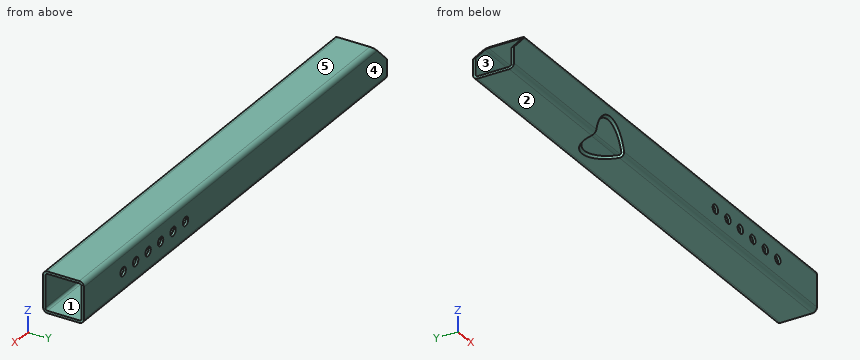
```python
from build123d import *

# Parameters (mm, degrees)
EL_MENT_M_CANO_SOUD_1_DEPTH = 850
ESQUISSE3_R                 = 7.5
ENL_V_MAT_EXTRU_2_DEPTH     = 90
ENL_V_MAT_EXTRU_3_DEPTH     = 71
ESQUISSE6_R                 = 40.75
ENL_V_MAT_EXTRU_4_DEPTH     = 90


with BuildPart() as part:
    # tube carré1 → Elément mécano-soudé1 (new body)
    with BuildSketch(Plane.YZ.offset(-425)):
        with BuildLine():
            Line((-27, 35), (27, 35))
            ThreePointArc((27, 35), (32.656854249, 32.656854249), (35, 27))
            Line((35, 27), (35, -27))
            ThreePointArc((35, -27), (32.656854249, -32.656854249), (27, -35))
            Line((27, -35), (-27, -35))
            ThreePointArc((-27, -35), (-32.656854249, -32.656854249), (-35, -27))
            Line((-35, -27), (-35, 27))
            ThreePointArc((-35, 27), (-32.656854249, 32.656854249), (-27, 35))
        make_face()
        with BuildLine():
            Line((-27, 31), (27, 31))
            ThreePointArc((27, 31), (29.828427336, 29.828426914), (31, 26.999999403))
            Line((31, 26.999999403), (31, -26.999999403))
            ThreePointArc((31, -26.999999403), (29.828427336, -29.828426914), (27, -31))
            Line((27, -31), (-27, -31))
            ThreePointArc((-27, -31), (-29.828427336, -29.828426914), (-31, -26.999999403))
            Line((-31, -26.999999403), (-31, 26.999999403))
            ThreePointArc((-31, 26.999999403), (-29.828427336, 29.828426914), (-27, 31))
        make_face(mode=Mode.SUBTRACT)
    extrude(amount=EL_MENT_M_CANO_SOUD_1_DEPTH)

    # Esquisse3 → Enlèv. mat.-Extru.2 (cut)
    with BuildSketch(Plane(origin=(0, 35, 0), x_dir=(1, 0, 0), z_dir=(0, 1, 0))):
        with Locations(Location((315, 0, 0), (0, 0, 270))):  # turned: the seam where the file's is
            Circle(ESQUISSE3_R)
        with Locations(Location((280, 0, 0), (0, 0, 270))):  # turned: the seam where the file's is
            Circle(ESQUISSE3_R)
        with Locations(Location((245, 0, 0), (0, 0, 270))):  # turned: the seam where the file's is
            Circle(ESQUISSE3_R)
        with Locations(Location((210, 0, 0), (0, 0, 270))):  # turned: the seam where the file's is
            Circle(ESQUISSE3_R)
        with Locations(Location((175, 0, 0), (0, 0, 270))):  # turned: the seam where the file's is
            Circle(ESQUISSE3_R)
        with Locations(Location((140, 0, 0), (0, 0, 270))):  # turned: the seam where the file's is
            Circle(ESQUISSE3_R)
    extrude(amount=-ENL_V_MAT_EXTRU_2_DEPTH, mode=Mode.SUBTRACT)

    # Esquisse5 → Enlèv. mat.-Extru.3 (cut, through all)
    with BuildSketch(Plane(origin=(0, 35, 0), x_dir=(1, 0, 0), z_dir=(0, 1, 0))):
        Polygon((-425, 0), (-390, -35), (-425, -35), align=None)
    extrude(amount=-ENL_V_MAT_EXTRU_3_DEPTH, mode=Mode.SUBTRACT)

    # Esquisse6 → Enlèv. mat.-Extru.4 (cut, symmetric)
    with BuildSketch(Plane(origin=(0, 2.000000299, -2.000000299), x_dir=(1, 0, 0), z_dir=(0, -0.707106781, 0.707106781))):
        with Locations((-155, -56.183766184)):
            Circle(ESQUISSE6_R)
    extrude(amount=ENL_V_MAT_EXTRU_4_DEPTH, both=True, mode=Mode.SUBTRACT)


solid = part.part
```
Here's how the part is built. I have some questions about the finished solid (model axes, mm). Face numbers are marked on the shaded views. A direction names the side the tool comes from. Give positions to 0.01 mm unless a question says otherwise; leave off trailing zeros. Write each loop counter-clockwise with the first axis right and the second up, starting at its lowest first coordinate (ties: lowest second). Pieces come first, ordered by that corner, then holes. Notation, with made-up numbers: M 29.5,50 L 81.5,50 A25 ccw 81.5,69 Z; hole C -30.75,75 d10. An arc over 180 degrees is marked long. Put each result on its own line as item: value. Start each with the question number.
Item 1: On a 3-axis mill with a long thin cutter (end or side, diameter ignored), from which of +Z, -Z, +X, -X, +Y, -Y can I reach the whole of each face in a straight line? I mean the marked faces 1 and 2. Say none if no direction works.
Item 2: If we section it at B-B, the plane x = -282: Write out the boundary of the cut face in (y, z), then the cut area to 3 significant figures.
Item 3: Will this pin go through, and if not, where does the flat tip stop? pin 1 (12 mm diameter, centred on x = 280, z = 0, fed in from +Y).
Item 4: If we section it at C-C, the plane z = -18: Count the separate pieces of the cut face and the enclosed holes in it, then the cut area to 3 significant figures.
Item 5: Thinking about a two-plate mould opening in Y: for the marked faces 3, 4 and 5, which applies, +Y half, -Y half, draft (parallel to the pull), parting line (faces both ways), or undercut?
Item 6: If we section it at A-A, the plane x = 210: Write out the boundary of the cut face in (y, z), then the cut area to 3 significant figures.
Item 7: I need wall thicknesses on L1, parallel to Z at x = -274, y = 1.5; L2, parallel to Z at x = -100, y = -30. Which ranges of each line are inside material? Lowest first, please. Write a range as from..to.
Values:
1. face 1: +X, -X
1. face 2: -Z, +X, -X, +Y, -Y
2. outline: M -35,-27 A8 ccw -27,-35 L 27,-35 A8 ccw 35,-27 L 35,27 A8 ccw 27,35 L -27,35 A8 ccw -35,27 Z; hole M -31,-27 A4 ccw -27,-31 L 27,-31 A4 ccw 31,-27 L 31,27 A4 ccw 27,31 L -27,31 A4 ccw -31,27 Z
2. area: 1,010 mm²
3. pin 1: through
4. separate pieces: 3
4. enclosed holes: 0
4. area: 6,520 mm²
5. face 3: undercut
5. face 4: +Y half
5. face 5: draft
6. outline: M -35,-27 A8 ccw -27,-35 L 27,-35 A8 ccw 35,-27 L 35,-7.5 L 31,-7.5 L 31,-27 A4 cw 27,-31 L -27,-31 A4 cw -31,-27 L -31,-7.5 L -35,-7.5 Z; M -35,7.5 L -31,7.5 L -31,27 A4 cw -27,31 L 27,31 A4 cw 31,27 L 31,7.5 L 35,7.5 L 35,27 A8 ccw 27,35 L -27,35 A8 ccw -35,27 Z
6. area: 895 mm²
7. L1: -35..-31, 31..35
7. L2: -34.42..-29.65, 29.65..34.42
